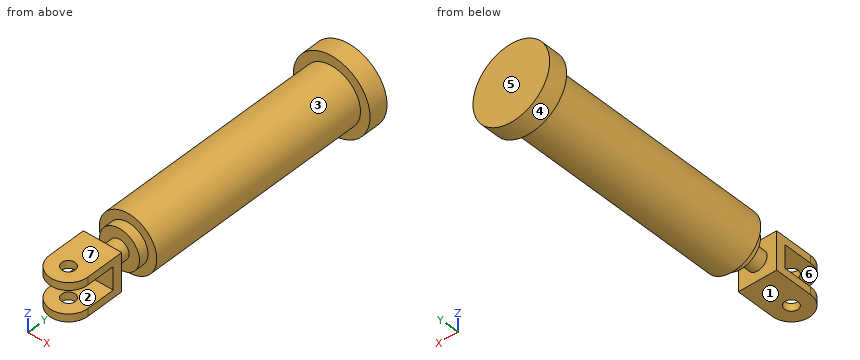
from build123d import *

# Parameters (mm, degrees)
SKETCH3_R           = 20
BOSS_EXTRUDE1_DEPTH = 10
SKETCH4_R           = 15
BOSS_EXTRUDE2_DEPTH = 120
SKETCH5_R           = 10.435871031
BOSS_EXTRUDE3_DEPTH = 5
SKETCH6_R           = 5
BOSS_EXTRUDE4_DEPTH = 10
SKETCH7_W           = 20
SKETCH7_H           = 20
BOSS_EXTRUDE5_DEPTH = 5
SKETCH8_R           = 3.5
BOSS_EXTRUDE6_DEPTH = 20
SKETCH9_W           = 12
SKETCH9_H           = 25
CUT_EXTRUDE1_DEPTH  = 27


with BuildPart() as part:
    # Sketch3 → Boss-Extrude1 (new body)
    with BuildSketch(Plane(origin=(0, 0, 0), x_dir=(1, 0, 0), z_dir=(0, 1, 0))):
        with Locations(Location((0, 0, 0), (0, 0, 270))):
            Circle(SKETCH3_R)
    extrude(amount=-BOSS_EXTRUDE1_DEPTH)

    # Sketch4 → Boss-Extrude2 (add)
    with BuildSketch(Plane.XZ.offset(10)):
        with Locations(Location((0, 0, 0), (0, 0, 270))):
            Circle(SKETCH4_R)
    extrude(amount=BOSS_EXTRUDE2_DEPTH)

    # Sketch5 → Boss-Extrude3 (add)
    with BuildSketch(Plane.XZ.offset(130)):
        with Locations(Location((0, 0, 0), (0, 0, 270))):
            Circle(SKETCH5_R)
    extrude(amount=BOSS_EXTRUDE3_DEPTH)

    # Sketch6 → Boss-Extrude4 (add)
    with BuildSketch(Plane(origin=(0, -135, 0), x_dir=(-1, 0, 0), z_dir=(0, -1, 0))):
        with Locations(Location((0, 0, 0), (0, 0, 90))):
            Circle(SKETCH6_R)
    extrude(amount=BOSS_EXTRUDE4_DEPTH)

    # Sketch7 → Boss-Extrude5 (add)
    with BuildSketch(Plane.XZ.offset(145)):
        Rectangle(SKETCH7_W, SKETCH7_H)
    extrude(amount=BOSS_EXTRUDE5_DEPTH)

    # Sketch8 → Boss-Extrude6 (add)
    with BuildSketch(Plane(origin=(0, 0, -10), x_dir=(-1, 0, 0), z_dir=(0, 0, -1))):
        with BuildLine():
            Line((-10, -150), (-10, -165))
            ThreePointArc((-10, -165), (0, -175), (10, -165))
            Line((10, -165), (10, -150))
            Line((10, -150), (-10, -150))
        make_face()
        with Locations((0, -165)):
            Circle(SKETCH8_R, mode=Mode.SUBTRACT)
    extrude(amount=-BOSS_EXTRUDE6_DEPTH)

    # Sketch9 → Cut-Extrude1 (cut, symmetric)
    with BuildSketch(Plane.ZY.offset(10)):
        with Locations((0, -162.5)):
            Rectangle(SKETCH9_W, SKETCH9_H)
    extrude(amount=CUT_EXTRUDE1_DEPTH, both=True, mode=Mode.SUBTRACT)


solid = part.part
Geometry: final body of the model. Coordinates: model frame, mm. Face numbers are marked on the shaded views. A direction names the side the tool comes from. Round coordinates to 2 decimals unless told otherwise and drop trailing zeros. Order: outer loops, then holes, each group sorted by start corner. A loop starts at its lowest first (then second) coordinate and runs counter-clockwise, first axis right, second up.
Q1. Access query for the marked faces 1, 2 and 3. Directions: +Z, -Z, +X, -X, +Y, -Y. A direction counts if a zero-diameter tool reaches every point of the face in a straight line with its end or side. Return the directions, or none.
Result sheet:
face 1: -Z, +X, -X, -Y
face 2: +X, -X, -Y
face 3: -Y
Q2. Section A-A, the plane x = 0. Give the number of separate pieces and of enclosed holes in the cut face, and give its area (3 significant figures).
Result sheet:
separate pieces: 3
enclosed holes: 0
area: 4,450 mm2
Q3. Section C-C, the plane x = -7. Output: boundary loops of the cut face in (y, z) (1 decimal), and give its area (3 significant figures).
Result sheet:
outline: (-172.1, -10) - (-145, -10) - (-145, 10) - (-172.1, 10) - (-172.1, 6) - (-150, 6) - (-150, -6) - (-172.1, -6) - close; (-135, -7.7) - (-130, -7.7) - (-130, -13.3) - (-10, -13.3) - (-10, -18.7) - (0, -18.7) - (0, 18.7) - (-10, 18.7) - (-10, 13.3) - (-130, 13.3) - (-130, 7.7) - (-135, 7.7) - close
area: 3,910 mm2
Q4. Material intervals for probe 1 along Y at (x, z) = (0, -8.4); probe 2 along X at (y, z) = (-165, 7); probe 3 along Y at (x, z) = (-4.5, -7.5), sorted ascending.
Result sheet:
probe 1: y = -175 to -168.5, -161.5 to -145, -135 to 0
probe 2: x = -10 to -3.5, 3.5 to 10
probe 3: y = -173.93 to -145, -135 to 0
Q5. Mould query, pull axis Z, two halves, no side actions, for the marked faces 4, 5, 6 and 7. Classes: released by +Z, released by -Z, zero draft, split by the parting line, or undercut.
Result sheet:
face 4: split by the parting line
face 5: zero draft
face 6: undercut
face 7: released by +Z
Q6. Section D-D, the plane y = -111. Output: boundary loops of the cut face in (x, z).
Result sheet:
outline: circle Ø30 at (0, 0)
Q7. Pin query (flat end, axial travel): pin 1 (16 mm diameter, centred on y = -159.5, z = 0.5, fed in from -X); pin 2 (16 mm diameter, centred on x = 1.5, y = -164.5, fed in from -Z); pin 3 (3 mm diameter, centred on x = 13.5, y = -19, fed in from +Z). Return the tip coordinate at first contact, or that it passes through.
Result sheet:
pin 1: stops at x = -10
pin 2: stops at z = -10
pin 3: stops at z = 9
Q8. Section B-B, the plane z = 0. Output: boundary loops of the cut face in (x, y).
Result sheet:
outline: (-20, -10) - (-15, -10) - (-15, -130) - (-10.44, -130) - (-10.44, -135) - (-5, -135) - (-5, -145) - (-10, -145) - (-10, -150) - (10, -150) - (10, -145) - (5, -145) - (5, -135) - (10.44, -135) - (10.44, -130) - (15, -130) - (15, -10) - (20, -10) - (20, 0) - (-20, 0) - close
